Here's how the part is built. I have some questions about the finished solid (model axes, mm). Coordinates: 2 decimals unless noted, no trailing zeros. Write each loop counter-clockwise with the first axis right and the second up, starting at its lowest first coordinate (ties: lowest second). Pieces come first, ordered by that corner, then holes. Notation, with made-up numbers: (-21, 88) -> (6, 88) arc R17 ccw to (6, 103) -> close; hole circle Ø11 at (29, 38). An arc over 180 degrees is marked (long way). Use a Markdown table: item, result. Add a question column.
Item 1: If I drill on line 1 along X through (y, z) = (-16.45, 7); line 2 along X through (y, z) = (-15.25, 50); line 3 along Z through (x, y) = (23, -16.4), over which ranges is the centre line in solid material (lowest first)? Write a range as from..to.
Item 2: Imagine slicing it at B-B, the plane y = -14.85. Write out the boundary of the cut face in (x, z).
Item 3: Imagine slicing it at D-D, the plane z = 53. Write out the boundary of the cut face in (x, y), and give its area (3 significant figures).
Item 4: Will these pins go through, and if not, where does the flat tip stop? pin 1 Ø1 at (x, y) = (22, -14.5) entering from -Z; pin 2 Ø9.5 at (x, z) = (29.5, 38) entering from -Y.
Item 5: Imagine slicing it at C-C, the plane x = 11.5. Write out the boundary of the cut face in (y, z).
Item 6: Imagine slicing it at A-A, the plane z = -2.5. Write out the boundary of the cut face in (x, y), and give its area (3 significant figures).
```python
from build123d import *

# Parameters (mm, degrees)
F2_DEPTH = 5
F5_DEPTH = 1.3
F7_R     = 6
F7_R_2   = 4.2
F8_DEPTH = 5.001
F9_R     = 2
F10_R    = 1


with BuildPart() as f2:
    # F1 (on offset) → F2 (new body)
    with BuildSketch(Plane.XZ.offset(13)):
        Polygon((17, 75), (7, 75), (7, -13), (18.8, -13), (18.8, 12), (27.2, 12), (27.2, -13), (39, -13), (39, 75), (29, 75), (29, 50), (17, 50), align=None)
    extrude(amount=F2_DEPTH)

    # F4 (on offset) → F5 (cut)
    with BuildSketch(Plane.XZ.offset(18)):
        Polygon((7, 16), (39, 16), (39, 75), (29, 75), (29, 50), (17, 50), (17, 75), (7, 75), align=None)
    extrude(amount=-F5_DEPTH, mode=Mode.SUBTRACT)

    # F7 (on offset) → F8 (cut, through all)
    with BuildSketch(Plane.XZ.offset(18)):
        with Locations((23, 50)):
            Circle(F7_R)
        with Locations((23, 12)):
            Circle(F7_R_2)
    extrude(amount=-F8_DEPTH, mode=Mode.SUBTRACT)

    # F9
    f9_edges = [f2.edges().sort_by_distance(p)[0] for p in [
        (7, -14.85, 75),
        (17, -14.85, 75),
        (29, -14.85, 75),
        (39, -14.85, 75),
        (7, -15.5, -13),
        (18.8, -15.5, -13),
        (27.2, -15.5, -13),
        (39, -15.5, -13),
    ]]
    fillet(f9_edges, radius=F9_R)

    # F10
    f10_edges = [f2.edges().sort_by_distance(p)[0] for p in [
        (21.719375, -17.35, 16),
        (24.280625, -17.35, 16),
    ]]
    fillet(f10_edges, radius=F10_R)


solid = f2.part
```
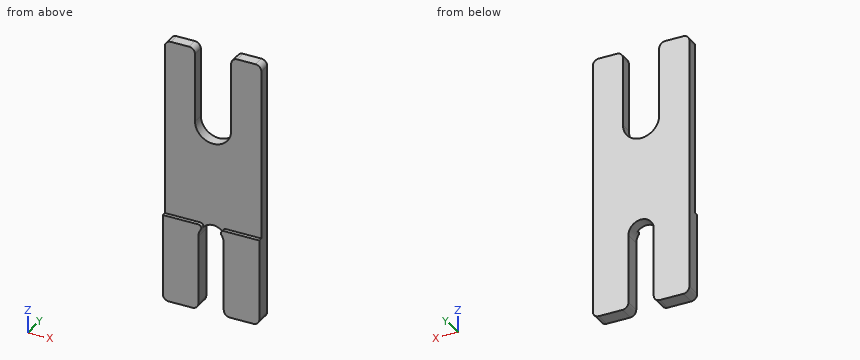
Ans:
| question | item | result |
|---|---|---|
| 1 | line 1 | x = 7..18.8, 27.2..39 |
| 1 | line 2 | x = 7..17, 29..39 |
| 1 | line 3 | z = 16.2..44 |
| 2 | outline | (7, -11) arc R2 ccw to (9, -13) -> (16.8, -13) arc R2 ccw to (18.8, -11) -> (18.8, 12) arc R4.2 cw to (27.2, 12) -> (27.2, -11) arc R2 ccw to (29.2, -13) -> (37, -13) arc R2 ccw to (39, -11) -> (39, 73) arc R2 ccw to (37, 75) -> (31, 75) arc R2 ccw to (29, 73) -> (29, 50) arc R6 cw to (17, 50) -> (17, 73) arc R2 ccw to (15, 75) -> (9, 75) arc R2 ccw to (7, 73) -> close |
| 3 | outline | (7, -16.7) -> (17, -16.7) -> (17, -13) -> (7, -13) -> close; (29, -16.7) -> (39, -16.7) -> (39, -13) -> (29, -13) -> close |
| 3 | area | 74.0 mm^2 |
| 4 | pin 1 | stops at z = 15.92 |
| 4 | pin 2 | stops at y = -16.7 |
| 5 | outline | (-18, -13) -> (-13, -13) -> (-13, 75) -> (-16.7, 75) -> (-16.7, 16) -> (-18, 16) -> close |
| 6 | outline | (7, -18) -> (18.8, -18) -> (18.8, -13) -> (7, -13) -> close; (27.2, -18) -> (39, -18) -> (39, -13) -> (27.2, -13) -> close |
| 6 | area | 118 mm^2 |
